Check sheet for the modelled part. Datum: model origin and axes. Units: mm. A direction names the side the tool comes from. Give positions to 0.01 mm unless a question says otherwise; leave off trailing zeros. Order: outer loops, then holes, each group sorted by start corner. A loop starts at its lowest first (then second) coordinate and runs counter-clockwise, first axis right, second up.
```python
from build123d import *

# Parameters (mm, degrees)
BOSS_EXTRUDE1_DEPTH = 10
SKETCH2_R           = 1
CUT_EXTRUDE1_DEPTH  = 23


with BuildPart() as part:
    # Sketch1 → Boss-Extrude1 (new body)
    with BuildSketch(Plane.XY):
        with BuildLine():
            Line((-13.971915032, 11), (17.028084968, 11))
            Line((17.028084968, 11), (12.841878076, 8))
            Line((12.841878076, 8), (8, 8))
            ThreePointArc((8, 8), (2.343145751, 5.656854249), (0, 0))
            Line((0, 0), (-7.971915032, 0))
            ThreePointArc((-7.971915032, 0), (-9.729274345, 4.242640687), (-13.971915032, 6))
            Line((-13.971915032, 6), (-13.971915032, 11))
        make_face()
    boss_extrude1 = extrude(amount=BOSS_EXTRUDE1_DEPTH)

    # Mirror1: Boss-Extrude1 across plane
    add(boss_extrude1.mirror(Plane.ZX))

    # Sketch2 → Cut-Extrude1 (cut, through all)
    with BuildSketch(Plane(origin=(0, 11, 0), x_dir=(1, 0, 0), z_dir=(0, 1, 0))):
        with Locations((-12.174520537, -5.224275734)):
            Circle(SKETCH2_R)
        with Locations((-2.174520537, -5.224275734)):
            Circle(SKETCH2_R)
    extrude(amount=-CUT_EXTRUDE1_DEPTH, mode=Mode.SUBTRACT)


solid = part.part
```
(1) Cross-section at C-C on y = 3.5. Enter the section's corners in (x, z).
Response values:
outline: (-9.1, 0) - (0.81, 0) - (0.81, 10) - (-9.1, 10) - close; hole circle Ø2 at (-2.17, 5.22)
(2) Cross-section at D-D on y = -6.5. Enter the section's corners in (x, z), then the cut area to 3 significant figures.
Response values:
outline: (-13.97, 0) - (3.34, 0) - (3.34, 10) - (-13.97, 10) - close; hole circle Ø2 at (-12.17, 5.22); hole circle Ø2 at (-2.17, 5.22)
area: 167 mm2
(3) Material ranges on L1, parallel to Y at x = 9.5, z = 6.25; L2, parallel to X at y = 8.5, z = 5.5; L3, parallel to X at y = -9.5, z = 4.5, recorded low to high.
Response values:
L1: y = -11 to -8, 8 to 11
L2: x = -13.97 to -13.14, -11.21 to -3.14, -1.21 to 13.54
L3: x = -13.97 to -12.86, -11.49 to -2.86, -1.49 to 14.93
(4) Cross-section at A-A on x = 5. Enter the section's corners in (y, z).
Response values:
outline: (-11, 0) - (-7.42, 0) - (-7.42, 10) - (-11, 10) - close; (7.42, 0) - (11, 0) - (11, 10) - (7.42, 10) - close
(5) Set-up check for faces 1 (the face through (10, -8, 5)), 2 (the face through (-13.972, 8, 5)): record each of +Z, -Z, +X, -X, +Y, -Y from which the full face is reachable in a straight line by a thin tool's end or side.
Response values:
face 1: +Z, -Z, +X
face 2: +Z, -Z, -X, +Y, -Y
(6) Cross-section at B-B on z = 8.75. Enter the section's corners in (x, y), then the cut area to 3 significant figures.
Response values:
outline: (-13.97, -11) - (17.03, -11) - (12.84, -8) - (8, -8) arc R8 cw to (8, 8) - (12.84, 8) - (17.03, 11) - (-13.97, 11) - (-13.97, 6) arc R6 cw to (-13.97, -6) - close
area: 368 mm2
(7) Gauge pin test, flat ends, axial feed: pin 1 Ø1 at (y, z) = (-0.5, 4.5) entering from -X; pin 2 Ø2 at (y, z) = (-8, 3) entering from +X; pin 3 Ø2 at (y, z) = (3, 7.5) entering from -X. Record the tip position at first contact, or that the pin passes through.
Response values:
pin 1: stops at x = -8.06
pin 2: stops at x = 14.24
pin 3: stops at x = -9.5
(8) Release check for a two-part mould opening along X. For faces 3 (the face through (-13.972, -8, 5)), 4 (the face through (-1.64, 0.15, 4.38)), 5 (the face through (10, 8, 5)), 6 (the face through (14.96, -9.52, 4.93)) record: released by +X, released by -X, zero draft, split by the parting line, or undercut.
Response values:
face 3: released by -X
face 4: undercut
face 5: zero draft
face 6: released by +X
